from build123d import *

# Parameters (mm, degrees)
ESQUISSE3_R        = 35
BOSS_EXTRU_3_DEPTH = 5


with BuildPart() as part:
    # Esquisse3 → Boss.-Extru.3 (new body)
    with BuildSketch(Plane(origin=(0, 0, 0), x_dir=(1, 0, 0), z_dir=(0, 1, 0))):
        with BuildLine():
            Line((-115, -25), (-25, -25))
            Line((-25, -25), (-24.99494949, -24.500051021))
            ThreePointArc((-24.99494949, -24.500051021), (-34.998214236, 0.353553761), (-24.494897428, 25))
            Line((-24.494897428, 25), (-25, 25))
            Line((-25, 25), (-115, 25))
            Line((-115, 25), (-115, -25))
        make_face()
        Circle(ESQUISSE3_R)
        Polygon((-9.403186381, -33.713203436), (35.849364905, -112.092921435), (79.150635095, -87.092921435), (34.150635095, -9.150635095), align=None)
        with BuildLine():
            Line((-24.494897428, 25), (-24.99494949, -24.500051021))
            ThreePointArc((-24.99494949, -24.500051021), (-17.805293657, -30.132565736), (-9.403186381, -33.713203436))
            Line((-9.403186381, -33.713203436), (33.715141323, -9.396235714))
            ThreePointArc((33.715141323, -9.396235714), (34.677297662, -4.741837919), (35, 0))
            ThreePointArc((35, 0), (34.72342821, 4.391302011), (33.898083809, 8.713203436))
            Line((33.898083809, 8.713203436), (-8.720191833, 33.896286735))
            ThreePointArc((-8.720191833, 33.896286735), (-17.19292058, 30.486119496), (-24.494897428, 25))
        make_face()
        Circle(ESQUISSE3_R)
        Polygon((33.898083809, 8.713203436), (79.150635095, 87.092921435), (35.849364905, 112.092921435), (-9.150635095, 34.150635095), align=None)
        with BuildLine():
            ThreePointArc((33.898083809, 8.713203436), (17.805293657, 30.132565736), (-8.720191833, 33.896286735))
            Line((-8.720191833, 33.896286735), (33.898083809, 8.713203436))
        make_face()
    extrude(amount=BOSS_EXTRU_3_DEPTH)


solid = part.part
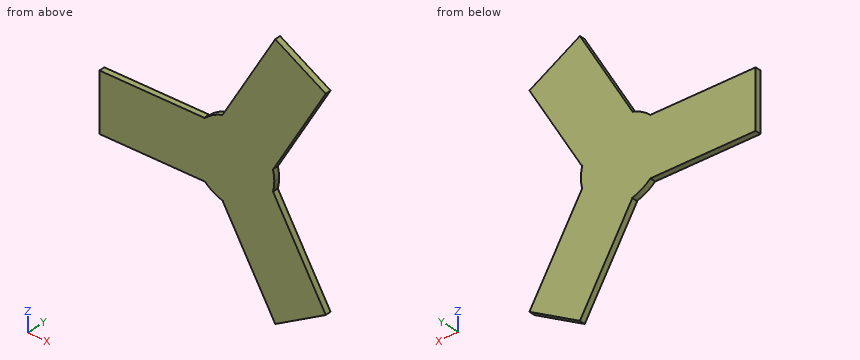
The listing builds one solid part. Answer for the finished solid, in the listing's coordinates (mm). Coordinates: 2 decimals unless noted, no trailing zeros. Write each loop counter-clockwise with the first axis right and the second up, starting at its lowest first coordinate (ties: lowest second). Pieces come first, ordered by that corner, then holes. Notation, with made-up numbers: (41, -6.5) - (64, -6.5) arc R14 ccw to (64, 4.5) - close; hole circle Ø3 at (84.5, 79.25). An arc over 180 degrees is marked (long way). Answer as CSV lines item,"result".
1. Given P1, Ø2.5, axis at x = -81.5, y = 2.5, coming from the -Z side; P2, Ø2, axis at x = -29.5, y = 3, coming from the +Z side; P3, Ø1.5, axis at y = 1, z = 57, coming from the +X side, each flat-ended and moving along its own axis, determine where each tip first touches the part or whether it passes through.
Computed values:
P1,"stops at z = -25"
P2,"stops at z = 25"
P3,"stops at x = 62.21"
2. Find section A-A (y = 2.9). Give the vertices of the cut face in (x, z), plus the area to 3 significant figures.
Computed values:
outline,"(-115, -25) - (-24.49, -25) arc R35 ccw to (-8.72, -33.9) - (-9.15, -34.15) - (35.85, -112.09) - (79.15, -87.09) - (33.9, -8.71) arc R35 ccw to (33.72, 9.4) - (34.15, 9.15) - (79.15, 87.09) - (35.85, 112.09) - (-9.4, 33.71) arc R35 ccw to (-24.99, 24.5) - (-25, 25) - (-115, 25) - close"
area,"16,300 mm²"
3. Find section D-D (z = -15.5). Give the vertices of the cut face in (x, y), plus the area to 3 significant figures.
Computed values:
outline,"(-115, 0) - (37.82, 0) - (37.82, 5) - (-115, 5) - close"
area,"764 mm²"
4. Straight lines are drawn through the part: line 1 (Z direction, x = 67, y = 2.8); line 2 (Z direction, x = 71.5, y = 0.75); line 3 (Z direction, x = -101.5, y = 1.25). For each, find the intervals that lie inside material, in ascending order. Write a range as [from, to].
Computed values:
line 1,"z = [-94.11, -66.05], [66.05, 94.11]"
line 2,"z = [-91.51, -73.84], [73.84, 91.51]"
line 3,"z = [-25, 25]"
5. Find section B-B (x = 65.5). Give the vertices of the cut face in (y, z).
Computed values:
outline,"(0, -94.97) - (5, -94.97) - (5, -63.45) - (0, -63.45) - close; (0, 63.45) - (5, 63.45) - (5, 94.97) - (0, 94.97) - close"
6. Find section C-C (x = -91.5). Give the vertices of the cut face in (y, z).
Computed values:
outline,"(0, -25) - (5, -25) - (5, 25) - (0, 25) - close"
